Autodesk Inventor part; units mm, degrees
ref_plane "YZ Plane" through (0, 0, 0) normal (1, 0, 0) x (0, 1, 0)
ref_plane "XZ Plane" through (0, 0, 0) normal (0, 1, 0) x (-1, 0, 0)
ref_plane "XY Plane" through (0, 0, 0) normal (0, 0, 1) x (1, 0, 0)
sketch "Sketch1" plane through (0, 0, 0) normal (0, 1, 0) x (-1, 0, 0)
  line L0 (-7.1438, -4.1244) -> (-7.1438, 4.1244)
  line L1 (-7.1438, 4.1244) -> (0, 8.2489)
  line L2 (0, 8.2489) -> (7.1438, 4.1244)
  line L3 (7.1438, 4.1244) -> (7.1437, -4.1244)
  line L4 (7.1437, -4.1244) -> (0, -8.2489)
  line L5 (0, -8.2489) -> (-7.1438, -4.1244)
  point P0 (0, 0)
  point P1 (0, 0)
  dimension "d0" = 14.2875
extrude "Extrusion1" add sketch "Sketch1" against normal blind 8.3344
sketch "Sketch2" plane through (0, 0, 0) normal (0, 1, 0) x (1, 0, 0)
  circle A0 centre (0, 0) radius 4.7625
  dimension "d3" = 9.525
extrude "Extrusion2" cut sketch "Sketch2" against normal through all
sketch "Sketch3" plane through (0, 0, 0) normal (1, 0, 0) x (0, 1, 0)
  line L0 (0, -4.7625) -> (-8.3344, -4.7625)
  line L1 (0, 4.7625) -> (0, -4.7625)
  line L2 (-10.188, 0) -> (2.7876, 0)
  line L3 (0, -4.7625) -> (-0.4986, -3.8989)
  line L4 (-0.4986, -3.8989) -> (-0.9972, -4.7625)
  point P0 (0, 0)
  dimension "d18" = 60
  dimension "d19" = 3.8989
  dimension "d20" = 30
coil "Coil2" sketch "Sketch3" operation add axis through (0, -10, 0) along (0, -1, 0) pitch 1.5875 turns 4.626 hand right
properties part number "boltExample"
Could you check a few things on this model? Use its own coordinates, in mm. A direction names the side the tool comes from. Round coordinates to 2 decimals unless told otherwise and drop trailing zeros. Order: outer loops, then holes, each group sorted by start corner. A loop starts at its lowest first (then second) coordinate and runs counter-clockwise, first axis right, second up.
(1) Which directions (+Z, -Z, +X, -X, +Y, -Y) give clear straight access to the entire face, cutting with the end or side of a thin tool? Please do faces 1 (the flat face through (3.62, -4.11, 6.16)), 2 (the flat face through (0, -0.5, -4.4)).
Response values:
face 1: +Z, +X, +Y, -Y
face 2: +Y
(2) I'm going to push flat-ended pins straight in: pin 1 (1 mm diameter, centred on x = -1.5, z = -1, fed in from -Y); pin 2 (2 mm diameter, centred on x = -1.5, y = -1.5, fed in from +Z); pin 3 (3 mm diameter, centred on x = 0, z = -3, fed in from -Y); pin 4 (8.5 mm diameter, centred on x = 0, z = 0, fed in from -Y). Where does each tip first touch, or does it pass through?
Response values:
pin 1: passes through
pin 2: stops at z = 7.96
pin 3: stops at y = -7.2
pin 4: stops at y = -8.05
(3) Please list where these lines run through material, in increasing order: line 1 along Y through (x, z) = (-6, -3.75); line 2 along X through (y, z) = (-2.95, 0); line 3 along X through (y, z) = (-8, 0.25).
Response values:
line 1: y = -8.33 to 0
line 2: x = -7.14 to -4.46, 4.71 to 7.14
line 3: x = -7.14 to -4.76, 4.76 to 7.14
(4) Imagine slicing it at A-A (z = -6). Write out the boundary of the cut face in (x, y), plus the area to 3 significant figures.
Response values:
outline: (-3.9, -8.33) - (3.9, -8.33) - (3.9, 0) - (-3.9, 0) - close
area: 64.9 mm2
(5) Imagine slicing it at B-B (x = -5.5). Write out the boundary of the cut face in (y, z).
Response values:
outline: (-8.33, -5.07) - (0, -5.07) - (0, 5.07) - (-8.33, 5.07) - close
